Input: part model. Units: mm. Frame: model coordinates. Face numbers are marked on the shaded views. A direction names the side the tool comes from. Round coordinates to 2 decimals unless told otherwise and drop trailing zeros. Loops run counter-clockwise (first coordinate to the right, second up) from the corner with the lowest first, then second, coordinate; pieces in that order, holes last. Notation, with made-up numbers: M -21.75,-16 L -4.75,-16 A17 cw -4.75,2 Z; hole C 78.25,89.5 d8. An arc over 180 degrees is marked long. Return JSON: item names as keys, results as strings. Group by question number.
1) Access query for the marked faces 1 and 2. Directions: +Z, -Z, +X, -X, +Y, -Y. A direction counts if a zero-diameter tool reaches every point of the face in a straight line with its end or side. Return the directions, or none.
2) Material intervals for line 1 (X direction, y = 10.5, z = -9); line 2 (Z direction, x = 44.5, y = -7.5); line 3 (Y direction, x = 57.5, z = 0), sorted ascending. Write a range as from..to.
3) Section B-B (x = 32). Output: boundary loops of the cut face in (y, z), plus the area to 3 significant figures.
4) Section A-A (x = 55.5). Output: boundary loops of the cut face in (y, z).
5) Contact query for flat-ended pins moving along their axis: P1, Ø0.8, axis at x = 4.5, y = -10, coming from the +Z side; P2, Ø0.8, axis at x = 5, y = -11, coming from the -Z side; P3, Ø6, axis at x = 38, y = 2.5, coming from the +Z side. Output: stop coordinate, or through.
from build123d import *
from build123d.topology import SkipClean

# Parameters (mm, degrees)
CHAMFER_1_SIZE      = 1.5
CHAMFER_2_SIZE      = 0.5
CUT_EXTRUDE_START   = -3
CUT_EXTRUDE_1_DEPTH = 3


# Read off the part's stored shape, not the designer's step: 切除-拉伸1
with BuildPart() as part:
    # 草图1 → 旋转1 (revolve)
    with BuildSketch(Plane.XY, mode=Mode.PRIVATE) as revolve_1_sk:
        Polygon((0, 0), (0, 12), (10, 12), (10, 11), (12, 11), (12, 12.5), (34, 12.5), (34, 15), (61, 15), (61, 17), (64, 17), (64, 0), align=None)
    revolve(revolve_1_sk.sketch.rotate(Axis((0, 0, 0), (-1, 0, 0)), 90), axis=Axis((0, 0, 0), (-1, 0, 0)))

    # 倒角1
    chamfer_1_edges = [part.edges().sort_by_distance(p)[0] for p in [
        (64, 0, 17),
    ]]
    chamfer(chamfer_1_edges, length=CHAMFER_1_SIZE)

    # 倒角2
    chamfer_2_edges = [part.edges().sort_by_distance(p)[0] for p in [
        (61, 0, 17),
        (34, 0, 15),
        (34, 0, 12.5),
        (12, 0, 12.5),
        (0, 0, 12),
    ]]
    chamfer(chamfer_2_edges, length=CHAMFER_2_SIZE)

    # 切除-拉伸1 outline → 切除-拉伸1 (cut)
    with SkipClean():  # the faces are left unmerged after this step: merging them gives an invalid solid
        with BuildSketch(Plane(origin=(0, -9, 0), x_dir=(1, 0, 0), z_dir=(0, 1, 0)).offset(CUT_EXTRUDE_START)):
            with BuildLine():
                Line((9.5, 2.5), (0, 2.5))
                Line((0, 2.5), (0, -2.5))
                Line((0, -2.5), (9.5, -2.5))
                ThreePointArc((9.5, -2.5), (12, 0), (9.5, 2.5))
            make_face()
        extrude(amount=CUT_EXTRUDE_1_DEPTH, mode=Mode.SUBTRACT)


solid = part.part
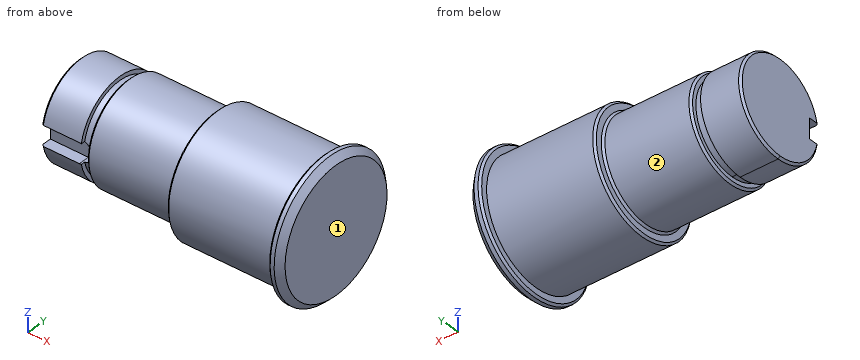
Returned:
{
 "1": {"face 1": "+Z, -Z, +X, +Y, -Y", "face 2": "-X"},
 "2": {"line 1": "x = 34..64", "line 2": "z = -12.99..12.99", "line 3": "y = -15..15"},
 "3": {"outline": "C 0,0 d25", "area": "491 mm^2"},
 "4": {"outline": "C 0,0 d30"},
 "5": {"P1": "stops at z = 7.2", "P2": "stops at z = -5.62", "P3": "stops at z = 15"}
}
